Here's how the part is built. I have some questions about the finished solid (model axes, mm). Face numbers are marked on the shaded views. A direction names the side the tool comes from. Give positions to 0.01 mm unless a question says otherwise; leave off trailing zeros. Loops run counter-clockwise (first coordinate to the right, second up) from the corner with the lowest first, then second, coordinate; pieces in that order, holes last. Notation, with made-up numbers: (40, 58) - (78, 58) arc R23 ccw to (78, 90) - close; hole circle Ø10 at (77, 14). An arc over 180 degrees is marked (long way). Return JSON: item names as keys, results as strings. Group by question number.
(1) For P1, Ø14, axis at x = 22, z = -22, coming from the -Y side; P2, Ø12, axis at y = 25, z = -5, coming from the -X side; P3, Ø3, axis at x = -6.5, y = 15.5, coming from the -Z side; P4, Ø20, axis at x = -9.5, y = 37, coming from the +Z side, each with a flat end and sliding along its axis, tell me the tip position at first contact or that it passes through.
(2) If we section it at B-B (z = 22): Please give me the cut outline in (x, y).
(3) If we section it at C-C (x = 0): Please give me the cut outline in (y, z), then the cut area to 3 significant figures.
(4) If we mould it in two halves opening along X, with no side actions, what happens to the marked faces 4, 5 and 6? For each: released by +X, released by -X, zero draft, split by the parting line, or undercut.
(5) I need wall thicknesses on probe 1 along X at (y, z) = (13, 65); probe 2 along X at (y, z) = (1, 0); probe 3 along Z at (x, y) = (-26.5, 39.5). Which ranges of each line are inside material? Lowest first, please. Write a range as [from, to].
(6) If we section it at D-D (x = 65): Please give me the cut outline in (y, z), then the cut area to 3 significant figures.
(7) On a 3-axis mill with a long thin cutter (end or side, diameter ignored), from which of +Z, -Z, +X, -X, +Y, -Y can I reach the whole of each face in a straight line? I mean the marked faces 1, 2 and 3. Say none if no direction works.
(8) If we section it at A-A (y = 15): State how many separate pieces and enclosed holes the cut face has, then the cut area to 3 significant figures.
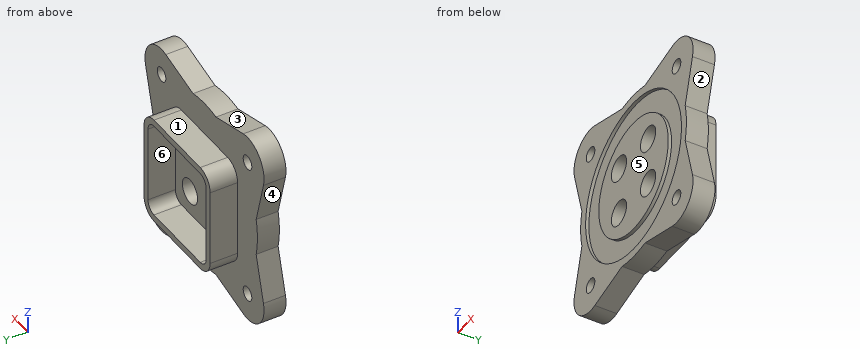
```python
from build123d import *

# Parameters (mm, degrees)
SKETCH1_R             = 11.5
BOSS_EXTRUDE1_DEPTH   = 20
SKETCH1_R_2           = 6.5
BOSS_EXTRUDE1_2_DEPTH = 20
BOSS_EXTRUDE2_DEPTH   = 45
SKETCH2_R             = 72.5
SKETCH2_R_2           = 52.5
CUT_EXTRUDE1_DEPTH    = 3


with BuildPart() as part:
    # Sketch1 → Boss-Extrude1 (new body)
    with BuildSketch(Plane(origin=(0, 0, 0), x_dir=(1, 0, 0), z_dir=(0, 1, 0))):
        with BuildLine():
            ThreePointArc((-44, 35), (-41.363961031, 41.363961031), (-35, 44))
            Line((-35, 44), (35, 44))
            ThreePointArc((35, 44), (41.363961031, 41.363961031), (44, 35))
            Line((44, 35), (44, -35))
            ThreePointArc((44, -35), (41.363961031, -41.363961031), (35, -44))
            Line((35, -44), (-35, -44))
            ThreePointArc((-35, -44), (-41.363961031, -41.363961031), (-44, -35))
            Line((-44, -35), (-44, 35))
        make_face()
        with Locations(Location((-22, 22, 0), (0, 0, 270))):
            Circle(SKETCH1_R, mode=Mode.SUBTRACT)
        with Locations(Location((22, 22, 0), (0, 0, 270))):
            Circle(SKETCH1_R, mode=Mode.SUBTRACT)
        with Locations(Location((-22, -22, 0), (0, 0, 270))):
            Circle(SKETCH1_R, mode=Mode.SUBTRACT)
        with Locations(Location((22, -22, 0), (0, 0, 270))):
            Circle(SKETCH1_R, mode=Mode.SUBTRACT)
    extrude(amount=BOSS_EXTRUDE1_DEPTH)



with BuildPart() as body_2:
    # Sketch1 → Boss-Extrude1 2 (new body)
    with BuildSketch(Plane(origin=(0, 0, 0), x_dir=(1, 0, 0), z_dir=(0, 1, 0))):
        with BuildLine():
            ThreePointArc((89.148145657, -58.529523872), (82.67766953, -82.67766953), (58.529523872, -89.148145657))
            Line((58.529523872, -89.148145657), (17.312897978, -78.104184034))
            ThreePointArc((17.312897978, -78.104184034), (0, -80), (-17.312897978, -78.104184034))
            Line((-17.312897978, -78.104184034), (-58.529523872, -89.148145657))
            ThreePointArc((-58.529523872, -89.148145657), (-82.67766953, -82.67766953), (-89.148145657, -58.529523872))
            Line((-89.148145657, -58.529523872), (-78.104184034, -17.312897978))
            ThreePointArc((-78.104184034, -17.312897978), (-80, 0), (-78.104184034, 17.312897978))
            Line((-78.104184034, 17.312897978), (-89.148145657, 58.529523872))
            ThreePointArc((-89.148145657, 58.529523872), (-82.67766953, 82.67766953), (-58.529523872, 89.148145657))
            Line((-58.529523872, 89.148145657), (-17.312897978, 78.104184034))
            ThreePointArc((-17.312897978, 78.104184034), (0, 80), (17.312897978, 78.104184034))
            Line((17.312897978, 78.104184034), (58.529523872, 89.148145657))
            ThreePointArc((58.529523872, 89.148145657), (82.67766953, 82.67766953), (89.148145657, 58.529523872))
            Line((89.148145657, 58.529523872), (78.104184034, 17.312897978))
            ThreePointArc((78.104184034, 17.312897978), (80, 0), (78.104184034, -17.312897978))
            Line((78.104184034, -17.312897978), (89.148145657, -58.529523872))
        make_face()
        with Locations(Location((65, -65, 0), (0, 0, 270))):
            Circle(SKETCH1_R_2, mode=Mode.SUBTRACT)
        with Locations(Location((-65, -65, 0), (0, 0, 270))):
            Circle(SKETCH1_R_2, mode=Mode.SUBTRACT)
        with Locations(Location((65, 65, 0), (0, 0, 270))):
            Circle(SKETCH1_R_2, mode=Mode.SUBTRACT)
        with Locations(Location((-65, 65, 0), (0, 0, 270))):
            Circle(SKETCH1_R_2, mode=Mode.SUBTRACT)
        with BuildLine():
            Line((-35, 50), (35, 50))
            ThreePointArc((35, 50), (45.606601718, 45.606601718), (50, 35))
            Line((50, 35), (50, -35))
            ThreePointArc((50, -35), (45.606601718, -45.606601718), (35, -50))
            Line((35, -50), (-35, -50))
            ThreePointArc((-35, -50), (-45.606601718, -45.606601718), (-50, -35))
            Line((-50, -35), (-50, 35))
            ThreePointArc((-50, 35), (-45.606601718, 45.606601718), (-35, 50))
        make_face(mode=Mode.SUBTRACT)
    extrude(amount=BOSS_EXTRUDE1_2_DEPTH)


with BuildPart() as part_1:
    add(part.part)

    add(body_2.part)  # Boss-Extrude2 merges body 2
    # Sketch1_3 → Boss-Extrude2 (add)
    with BuildSketch(Plane(origin=(0, 0, 0), x_dir=(1, 0, 0), z_dir=(0, 1, 0))):
        with BuildLine():
            ThreePointArc((35, 50), (45.606601718, 45.606601718), (50, 35))
            Line((50, 35), (50, -35))
            ThreePointArc((50, -35), (45.606601718, -45.606601718), (35, -50))
            Line((35, -50), (-35, -50))
            ThreePointArc((-35, -50), (-45.606601718, -45.606601718), (-50, -35))
            Line((-50, -35), (-50, 35))
            ThreePointArc((-50, 35), (-45.606601718, 45.606601718), (-35, 50))
            Line((-35, 50), (35, 50))
        make_face()
        with BuildLine():
            Line((-44, -35), (-44, 35))
            ThreePointArc((-44, 35), (-41.363961031, 41.363961031), (-35, 44))
            Line((-35, 44), (35, 44))
            ThreePointArc((35, 44), (41.363961031, 41.363961031), (44, 35))
            Line((44, 35), (44, -35))
            ThreePointArc((44, -35), (41.363961031, -41.363961031), (35, -44))
            Line((35, -44), (-35, -44))
            ThreePointArc((-35, -44), (-41.363961031, -41.363961031), (-44, -35))
        make_face(mode=Mode.SUBTRACT)
    extrude(amount=BOSS_EXTRUDE2_DEPTH)

    # Sketch2 → Cut-Extrude1 (cut)
    with BuildSketch(Plane.XZ):
        with Locations(Location((0, 0, 0), (0, 0, 270))):
            Circle(SKETCH2_R)
        with Locations(Location((0, 0, 0), (0, 0, 270))):
            Circle(SKETCH2_R_2, mode=Mode.SUBTRACT)
    extrude(amount=-CUT_EXTRUDE1_DEPTH, mode=Mode.SUBTRACT)


solid = part_1.part
```
Values:
{
 "1": {"P1": "through", "P2": "x = -79.98", "P3": "z = -79.84", "P4": "z = 50"},
 "2": {"outline": "(-79.36, 0) - (-69.08, 0) - (-69.08, 3) - (-47.67, 3) - (-47.67, 0) - (-33.5, 0) - (-33.5, 20) - (-44, 20) - (-44, 45) - (-50, 45) - (-50, 20) - (-79.36, 20) - close; (-10.5, 0) - (10.5, 0) - (10.5, 20) - (-10.5, 20) - close; (33.5, 0) - (47.67, 0) - (47.67, 3) - (69.08, 3) - (69.08, 0) - (79.36, 0) - (79.36, 20) - (50, 20) - (50, 45) - (44, 45) - (44, 20) - (33.5, 20) - close"},
 "3": {"outline": "(0, -80) - (20, -80) - (20, -50) - (45, -50) - (45, -44) - (20, -44) - (20, 44) - (45, 44) - (45, 50) - (20, 50) - (20, 80) - (0, 80) - (0, 72.5) - (3, 72.5) - (3, 52.5) - (0, 52.5) - (0, -52.5) - (3, -52.5) - (3, -72.5) - (0, -72.5) - close", "area": "3,380 mm2"},
 "4": {"face 4": "released by -X", "face 5": "zero draft", "face 6": "undercut"},
 "5": {"probe 1": "[-90, -71.5], [-58.5, 58.5], [71.5, 90]", "probe 2": "[-80, -72.5], [-52.5, 52.5], [72.5, 80]", "probe 3": "[-50, -44], [44, 50]"},
 "6": {"outline": "(0, -90) - (20, -90) - (20, -71.5) - (0, -71.5) - close; (0, -58.5) - (20, -58.5) - (20, 58.5) - (0, 58.5) - (0, 32.11) - (3, 32.11) - (3, -32.11) - (0, -32.11) - close; (0, 71.5) - (20, 71.5) - (20, 90) - (0, 90) - close", "area": "2,890 mm2"},
 "7": {"face 1": "+Z, +X, -X, +Y", "face 2": "+X, +Y, -Y", "face 3": "+Z, +Y, -Y"},
 "8": {"separate pieces": "1", "enclosed holes": "8", "area": "26,100 mm2"}
}
